```python
from build123d import *

# Parameters (mm, degrees)
SKETCH1_W            = 111.125
SKETCH1_H            = 85.725
BOSS_EXTRUDE1_DEPTH  = 3.175
M3_CLEARANCE_HOLE1_D = 4.5
M3_CLEARANCE_HOLE2_D = 4.5


with BuildPart() as part:
    # Sketch1 → Boss-Extrude1 (new body)
    with BuildSketch(Plane(origin=(0, 0, 0), x_dir=(1, 0, 0), z_dir=(0, 1, 0))):
        Rectangle(SKETCH1_W, SKETCH1_H)
    extrude(amount=BOSS_EXTRUDE1_DEPTH)

    # M3 Clearance Hole1 (through all)
    with Locations(Plane(origin=(-50.8, 0, 38.1), x_dir=(0, 0, -1), z_dir=(0, -1, 0))):
        with Locations((0, 0), (0, 101.6), (76.2, 0), (76.2, 101.6)):
            Hole(M3_CLEARANCE_HOLE1_D / 2)

    # M3 Clearance Hole2 (through all)
    with Locations(Plane(origin=(-29.5, 3.175, 36.5125), x_dir=(0, 0, 1), z_dir=(0, 1, 0))):
        with Locations((0, 0), (-24, 0), (-24, 59), (0, 59), (-38.025, 64), (-73.025, 64), (-73.025, -5), (-38.025, -5)):
            Hole(M3_CLEARANCE_HOLE2_D / 2)


solid = part.part
```
The listing builds one solid part. Answer for the finished solid, in the listing's coordinates (mm). Give positions to 0.01 mm unless a question says otherwise; leave off trailing zeros. Order: outer loops, then holes, each group sorted by start corner. A loop starts at its lowest first (then second) coordinate and runs counter-clockwise, first axis right, second up. Notation, with made-up numbers: (-16, -4) -> (20, -4) arc R30 cw to (20, 26) -> close; hole circle Ø4 at (85.5, -4). An arc over 180 degrees is marked (long way). Answer as CSV lines item,"result". Start each with the question number.
Q1. Given pin 1 (3.5 mm diameter, centred on x = 29.5, z = 36.51, fed in from +Y), flat-ended and moving along its own axis, determine where the tip first touches the part or whether it passes through.
Q2. Find the intervals of material crossed by L1, parallel to Z at x = 51.5, y = 0.6; L2, parallel to X at y = 2.55, z = 35; L3, parallel to Z at x = 49, y = 0.9, in increasing order.
Q3. A cutting plane is placed at A-A (x = -34.5). Determine the outline of the cut face in (y, z) (1 decimal).
Q4. A cutting plane is placed at C-C (z = 37). Determine the outline of the cut face in (x, y) (1 decimal), then the cut area to 3 significant figures.
Q5. A cutting plane is placed at B-B (y = 2.4). Count the separate pieces of the cut face and the enclosed holes in it, then the cut area to 3 significant figures.
Q6. Determine the mould class of faces 1 (the cylindrical face through (-50.124, 1.61, -35.954)), 2 (the flat face through (-55.562, 2, 1)), 3 (the flat face through (-1, 2, -42.862)) for opening direction Z: pulls with the +Z half, pulls with the -Z half, needs draft (parallel to the pull), parting line crosses it, or undercut.
Results found:
1,pin 1,"through"
2,L1,"-42.86 to -40.24, -35.96 to 35.96, 40.24 to 42.86"
2,L2,"-55.56 to -31.17, -27.83 to 27.83, 31.17 to 55.56"
2,L3,"-42.86 to -39.45, -36.75 to 36.75, 39.45 to 42.86"
3,outline,"(0, -42.9) -> (3.2, -42.9) -> (3.2, -38.8) -> (0, -38.8) -> close; (0, -34.3) -> (3.2, -34.3) -> (3.2, -3.8) -> (0, -3.8) -> close; (0, 0.7) -> (3.2, 0.7) -> (3.2, 42.9) -> (0, 42.9) -> close"
4,outline,"(-55.6, 0) -> (-52.8, 0) -> (-52.8, 3.2) -> (-55.6, 3.2) -> close; (-48.8, 0) -> (-31.7, 0) -> (-31.7, 3.2) -> (-48.8, 3.2) -> close; (-27.3, 0) -> (27.3, 0) -> (27.3, 3.2) -> (-27.3, 3.2) -> close; (31.7, 0) -> (48.8, 0) -> (48.8, 3.2) -> (31.7, 3.2) -> close; (52.8, 0) -> (55.6, 0) -> (55.6, 3.2) -> (52.8, 3.2) -> close"
4,area,"300 mm2"
5,separate pieces,"1"
5,enclosed holes,"12"
5,area,"9,340 mm2"
6,face 1,"undercut"
6,face 2,"needs draft"
6,face 3,"pulls with the -Z half"
